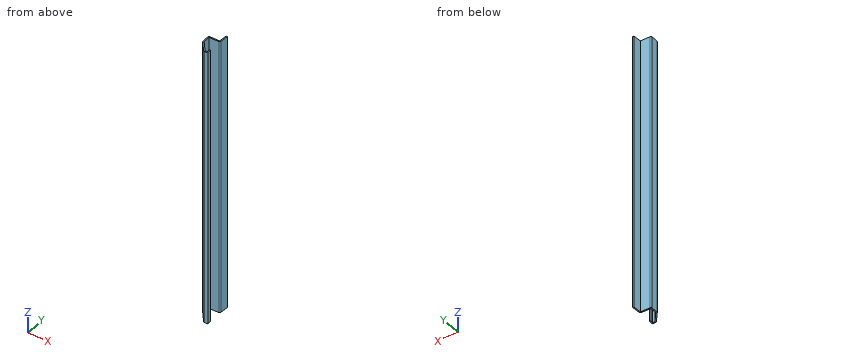
from build123d import *

# Parameters (mm, degrees)
EXTRUDE_THIN1_DEPTH = 206.375
FILLET1_R           = 0.889


with BuildPart() as part:
    # Sketch1 → Extrude-Thin1 (new body)
    with BuildSketch(Plane.XY):
        Polygon((-0.396875, 3.175), (0, 0), (-3.175, 0), (-9.525, 7.9375), (-9.525, 14.2875), (-1.285875, 14.2875), (-0.889, 20.6375), (-0.001731258, 20.582045704), (-0.450702864, 13.3985), (-8.636, 13.3985), (-8.636, 8.249344362), (-2.747724511, 0.889), (-1.007043392, 0.889), (-1.279010032, 3.064733121), align=None)
    extrude(amount=-EXTRUDE_THIN1_DEPTH)

    # Fillet1
    fillet1_edges = [part.edges().sort_by_distance(p)[0] for p in [
        (-0.450702864, 13.3985, -103.1875),
        (-3.175, 0, -103.1875),
        (-9.525, 7.9375, -103.1875),
        (-9.525, 14.2875, -103.1875),
    ]]
    fillet(fillet1_edges, radius=FILLET1_R)


solid = part.part
Check sheet for the modelled part. Datum: model origin and axes. Units: mm. Give positions to 0.01 mm unless a question says otherwise; leave off trailing zeros. Loops run counter-clockwise (first coordinate to the right, second up) from the corner with the lowest first, then second, coordinate; pieces in that order, holes last. Notation, with made-up numbers: M 71,81 L 121,81 A15 ccw 121,95 Z; hole C 45,33.25 d7. An arc over 180 degrees is marked long. Answer as a JSON object with one key per item and string values. Group by question number.
Q1. Material ranges on line 1 along Y through (x, z) = (-3.75, -179.5); line 2 along Y through (x, z) = (-7.25, -144); line 3 along X through (y, z) = (14.5, -99.5), recorded low to high. Write a range as [from, to].
Q2. Cross-section at B-B on z = -133.5. Record the cut outline in (x, y) (1 decimal), then the cut area to 3 significant figures.
Q3. Cross-section at C-C on y = 16.5. Record the cut outline in (x, z) (3 decimals).
Q4. Cross-section at A-A on x = -5.75. Record the cut outline in (y, z) (1 decimal), then the cut area to 3 significant figures.
Q5. Go/stop test with flat-tipped pins: P1, Ø1, axis at y = 7.5, z = -40, coming from the -X side; P2, Ø2, axis at y = 17, z = -159, coming from the -X side; P3, Ø1, axis at x = -4.5, z = -138.5, coming from the -Y side; P4, Ø1.5, axis at x = -3, y = 16.5, coming from the -Z side. Record where each tip stops, or that it passes through.
Evaluation:
{
 "1": {"line 1": "y = [0.72, 2.14], [13.4, 14.29]", "line 2": "y = [5.09, 6.52], [13.4, 14.29]", "line 3": "x = [-1.27, -0.38]"},
 "2": {"outline": "M -9.5,8.2 A0.9 ccw -9.3,7.7 L -3.4,0.3 A0.9 ccw -2.7,0 L 0,0 L -0.4,3.2 L -1.3,3.1 L -1,0.9 L -2.7,0.9 L -8.6,8.2 L -8.6,13.4 L -1.3,13.4 A0.9 ccw -0.4,14.2 L 0,20.6 L -0.9,20.6 L -1.3,14.3 L -8.6,14.3 A0.9 ccw -9.5,13.4 Z", "area": "31.4 mm2"},
 "3": {"outline": "M -1.148,-206.375 L -0.257,-206.375 L -0.257,0 L -1.148,0 Z"},
 "4": {"outline": "M 3.2,-206.4 L 4.6,-206.4 L 4.6,0 L 3.2,0 Z; M 13.4,-206.4 L 14.3,-206.4 L 14.3,0 L 13.4,0 Z", "area": "477 mm2"},
 "5": {"P1": "stops at x = -9.49", "P2": "stops at x = -1.18", "P3": "stops at y = 1.03", "P4": "passes through"}
}
